Autodesk Inventor part; units mm, degrees
ref_plane "Work Plane1" through (0, 0, -60) normal (0, 0, -1) x (-1, 0, 0)
ref_plane "YZ Plane" through (0, 0, 0) normal (1, 0, 0) x (0, 1, 0)
ref_plane "XZ Plane" through (0, 0, 0) normal (0, 1, 0) x (-1, 0, 0)
sketch "Sketch1" plane through (0, 0, 0) normal (0, 0, 1) x (1, 0, 0)
  arc A0 (-55, 0) -> (55, 0) centre (0, 0) ccw
  arc A1 (-70, 0) -> (63.2456, -30) centre (0, 0) ccw
  arc A2 (85, 0) -> (155, 0) centre (120, 0) ccw
  arc A3 (80, -30) -> (167.697, -15) centre (120, 0) ccw
  arc A4 (195, 0) -> (265, 0) centre (230, 0) ccw
  arc A5 (182.303, -15) -> (277.697, -15) centre (230, 0) ccw
  line L0 (-130, 0) -> (-130, -15)
  line L1 (310, -15) -> (310, 0)
  line L2 (-130, -15) -> (-68.374, -15)
  line L3 (-130, 0) -> (-55, 0)
  line L4 (63.2456, -30) -> (80, -30)
  line L5 (167.697, -15) -> (182.303, -15)
  line L6 (277.697, -15) -> (310, -15)
  line L7 (265, 0) -> (310, 0)
  line L8 (55, 0) -> (85, 0)
  line L9 (155, 0) -> (195, 0)
  line L10 (-88.374, -15) -> (-88.374, -145)
  line L11 (-88.374, -145) -> (291.626, -145)
  line L12 (291.626, -145) -> (291.626, -15)
  dimension "d0" = 110
  dimension "d1" = 140
  dimension "d2" = 70
  dimension "d3" = 100
  dimension "d4" = 70
  dimension "d5" = 100
  dimension "d8" = 440
  dimension "d9" = 130
  dimension "d10" = 15
  dimension "d12" = 130
  dimension "d13" = 380
  dimension "d14" = 20
extrude "Extrusion1" add sketch "Sketch1" along normal blind 30 contours A0 L8 A2 L9 A4 L7 L1 L6 A5 L5 A3 L4 A1 L3 | A1 L2 L0 L3
extrude "Extrusion2" add sketch "Sketch1" along normal blind 10 contours A1 L4 A3 L5 A5 L6 L12 L11 L10 L2
sketch "Sketch2" plane through (0, 0, 0) normal (0, 0, -1) x (-1, 0, 0)
  line L0 (-291.626, -145) -> (-291.626, -15)
  line L1 (88.374, -145) -> (-291.626, -145)
  line L2 (88.374, -15) -> (88.374, -145)
  line L3 (-281.626, -15) -> (-281.626, -135)
  line L4 (-281.626, -135) -> (78.374, -135)
  line L5 (78.374, -135) -> (78.374, -15)
  line L6 (-291.626, -15) -> (-310, -15)
  line L7 (130, -15) -> (88.374, -15)
  line L8 (-291.626, -15) -> (-281.626, -15)
  line L9 (78.374, -15) -> (88.374, -15)
  point P0 (0, 0)
  dimension "d19" = 10
extrude "Extrusion3" add sketch "Sketch2" along normal blind 130
ref_plane "Work Plane1" through (0, 0, -60) normal (0, 0, -1) x (-1, 0, 0)
mirror "Mirror1" about plane through (0, 0, -60) normal (0, 0, -1) of "Extrusion1", "Extrusion2"
sketch "Sketch3" plane through (0, 0, -60) normal (0, 0, -1) x (-1, 0, 0)
  line L0 (78.374, -135) -> (78.374, -15)
  line L1 (130, 0) -> (130, -15)
  line L2 (78.374, -15) -> (130, -15)
  line L3 (130, -15) -> (130, 0)
  line L4 (130, 0) -> (78.374, 0)
  line L5 (78.374, 0) -> (78.374, -15)
  line L6 (-281.626, -15) -> (-281.626, -135)
  line L7 (-310, 0) -> (-265, 0)
  line L8 (-281.626, -15) -> (-310, -15)
  line L9 (-310, -15) -> (-310, 0)
  line L10 (-310, 0) -> (-281.626, 0)
  line L11 (-281.626, 0) -> (-281.626, -15)
  point P0 (0, 0)
extrude "Extrusion4" add sketch "Sketch3" along normal through all both and the other way through all
sketch "Sketch4" plane through (0, 0, -60) normal (0, 0, -1) x (-1, 0, 0)
  line L0 (-291.626, -15) -> (-291.626, -145)
  line L1 (-343.586, -145) -> (141.414, -145)
  line L2 (141.414, -145) -> (141.414, -160)
  line L3 (141.414, -160) -> (-343.586, -160)
  line L4 (-343.586, -145) -> (-343.586, -160)
  point P0 (0, 0)
  dimension "d29" = 51.96
  dimension "d30" = 485
  dimension "d31" = 15
extrude "Extrusion5" add sketch "Sketch4" along normal mid plane 230
fillet "Fillet1" radius 10 6 edges at (0, -55, 30) (120, -35, 30) (230, -35, 30) (230, -35, -150) (120, -35, -150) (0, -55, -150)
sketch "Sketch5" plane through (-130, -15, 30) normal (0, -1, 0) x (1, 0, 0)
  point P0 (10, -10)
hole "Hole1" at (-120, -15, 20) direction (0, 1, 0) diameter 11 depth 15
sketch "Sketch6" plane through (-130, -15, 30) normal (0, -1, 0) x (1, 0, 0)
  point P0 (10, -170)
hole "Hole2" at (-120, -15, -140) direction (0, 1, 0) diameter 11 depth 15
sketch "Sketch7" plane through (277.697, -15, 30) normal (0, -1, 0) x (1, 0, 0)
  point P0 (22.303, -10)
hole "Hole3" at (300, -15, 20) direction (0, 1, 0) diameter 11 depth 15
sketch "Sketch8" plane through (277.697, -15, 30) normal (0, -1, 0) x (1, 0, 0)
  point P0 (22.303, -170)
hole "Hole4" at (300, -15, -140) direction (0, 1, 0) diameter 11 depth 15
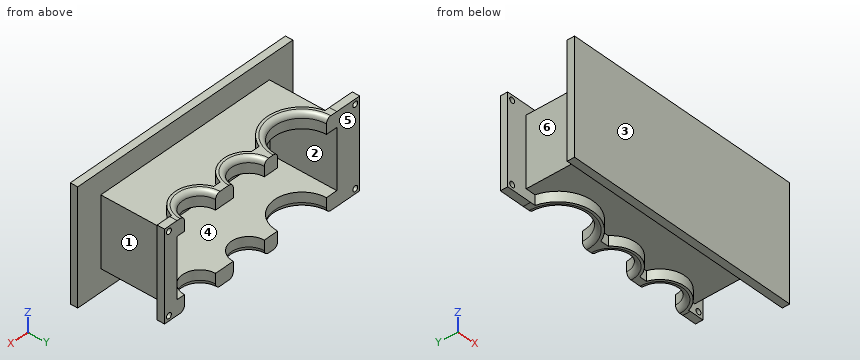
CAD build for the part. Positions are in the model's coordinates, mm. Face numbers are marked on the shaded views. A direction names the side the tool comes from. Coordinates: 2 decimals unless noted, no trailing zeros. Order: outer loops, then holes, each group sorted by start corner. A loop starts at its lowest first (then second) coordinate and runs counter-clockwise, first axis right, second up. Notation, with made-up numbers: (-28.5, -16) - (-0.5, -16) arc R13 cw to (-0.5, 5) - close; hole circle Ø1 at (-39.5, 2.5). An arc over 180 degrees is marked (long way). Use a Markdown table: item, result. Add a question column.
(1) Saw through at D-D (x = 230). Give the cut face in (y, z), then the cut area to 3 significant figures.
(2) Saw through at C-C (z = -78.5). Give the cut face in (x, y), then the cut area to 3 significant figures.
(3) Flat gauge pins, fed straight in: pin 1 (16.5 mm diameter, centred on x = -113, y = -10, fed in from +Z); pin 2 (16.5 mm diameter, centred on y = -6.5, z = -56, fed in from +X); pin 3 (10 mm diameter, centred on x = 143.5, z = -112.5, fed in from +Y); pin 4 (14.5 mm diameter, centred on x = -120, z = -140, fed in from +Y). Where does each tip first touch, or does it go through?
(4) Saw through at A-A (x = 300). Give the cut face in (y, z), then the cut area to 3 significant figures.
(5) Which spindle directions (+Z, -Z, +X, -X, +Y, -Y) get a long thin tool onto all of the face, cutting with end or side? Do the marked faces 5 and 6. Say none if no direction does.
(6) Saw through at B-B (y = -118). Give the cut face in (x, z).
(7) Pull direction X, two halves, no side cores. Call the marked faces 1, 2, 3 and 4: +X half, -X half, draft (parallel to the pull), parting line (faces both ways), or undercut.
(8) Drill centre lines: line 1 along Z through (x, y) = (-120, -8); line 2 along X through (y, z) = (-134.5, -108); line 3 along X through (y, z) = (-3, 20). Where is each one in solid material? Low to high. Write a range as [from, to].
Solved:
| question | item | result |
|---|---|---|
| 1 | outline | (-160, -175) - (-145, -175) - (-145, -130) - (-50, -130) - (-50, -150) - (-45, -150) arc R10 ccw to (-35, -140) - (-35, -120) - (-135, -120) - (-135, 0) - (-35, 0) - (-35, 20) arc R10 ccw to (-45, 30) - (-50, 30) - (-50, 10) - (-145, 10) - (-145, 55) - (-160, 55) - close |
| 1 | area | 7,410 mm² |
| 2 | outline | (-141.41, -160) - (343.59, -160) - (343.59, -145) - (291.63, -145) - (291.63, -15) - (310, -15) - (310, 0) - (281.63, 0) - (281.63, -135) - (-78.37, -135) - (-78.37, 0) - (-130, 0) - (-130, -15) - (-88.37, -15) - (-88.37, -145) - (-141.41, -145) - close |
| 2 | area | 14,700 mm² |
| 3 | pin 1 | stops at z = 30 |
| 3 | pin 2 | stops at x = 310 |
| 3 | pin 3 | stops at y = -135 |
| 3 | pin 4 | stops at y = 0 |
| 4 | outline | (-160, -175) - (-145, -175) - (-145, 55) - (-160, 55) - close; (-15, -150) - (0, -150) - (0, -145.5) - (-15, -145.5) - close; (-15, -134.5) - (0, -134.5) - (0, 14.5) - (-15, 14.5) - close; (-15, 25.5) - (0, 25.5) - (0, 30) - (-15, 30) - close |
| 4 | area | 5,820 mm² |
| 5 | face 5 | +Z, -Z, +X, -X, +Y |
| 5 | face 6 | +Z, -Z, -X |
| 6 | outline | (-88.37, -130) - (291.63, -130) - (291.63, 10) - (-88.37, 10) - close; hole (-78.37, -120) - (281.63, -120) - (281.63, 0) - (-78.37, 0) - close |
| 7 | face 1 | +X half |
| 7 | face 2 | undercut |
| 7 | face 3 | draft |
| 7 | face 4 | undercut |
| 8 | line 1 | z = [-150, -145.5], [-134.5, 14.5], [25.5, 30] |
| 8 | line 2 | x = [-88.37, -78.37], [281.63, 291.63] |
| 8 | line 3 | x = [-130, -125.5], [-114.5, -54.92], [54.92, 85.13], [154.87, 195.13], [264.87, 294.5], [305.5, 310] |
